Drawing for the job (mm, zero at the part's lowest x, y, z). Coordinates: 2 decimals unless noted, no trailing zeros. Write each loop counter-clockwise with the first axis right and the second up, starting at its lowest first coordinate (ties: lowest second). Pieces come first, ordered by that corner, then holes. Notation, with made-up numbers: M 52.5,69 L 75.5,69 A25 cw 75.5,84 Z; hole C 23,35 d1. An arc over 180 degrees is marked long. Put each result on its own line as item: value. Start each with the question number.
Q1. Drill centre lines: line 1 along X through (y, z) = (14.5, 0.7) (3 decimals); line 2 along Y through (x, z) = (20, 0.45); line 3 along Y through (x, z) = (30.5, 0.7). Where is each one in solid material? Low to high.
Q2. Cut at D-D (x = 23.5). Write the cut outline in (y, z), then the cut area to 3 significant figures.
Q3. Cut at C-C (x = 12.5). Write the cut outline in (y, z), then the cut area to 3 significant figures.
Q4. Cut at B-B (z = 0.35). Write the cut outline in (x, y) (3 decimals).
Q5. Cut at A-A (y = 21.5). Write the cut outline in (x, z) (3 decimals), then the cut area to 4 significant figures.
Q6. Drop flat-ended pins along their axis: pin 1 (0.8 mm diameter, centred on y = 15, z = 1, fed in from +X); pin 2 (0.8 mm diameter, centred on x = 40, z = 0.5, fed in from -Y). Give the stop position or say it passes through.
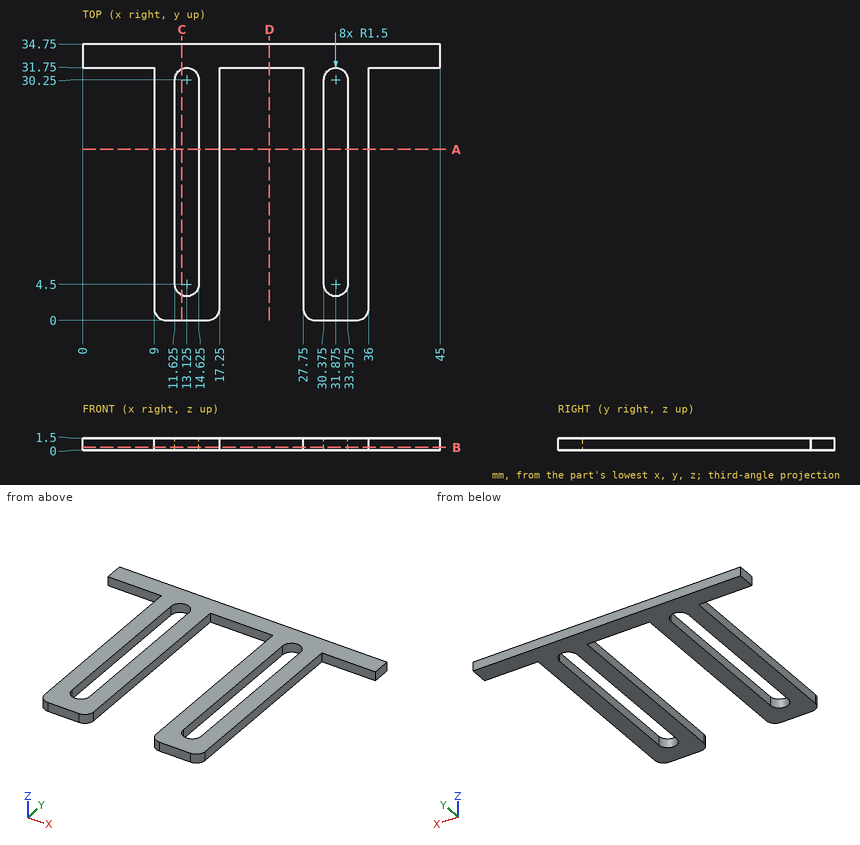
Computed values:
1. line 1: 9 to 11.625, 14.625 to 17.25, 27.75 to 30.375, 33.375 to 36
1. line 2: 31.75 to 34.75
1. line 3: 0 to 3.9, 30.85 to 34.75
2. outline: M 31.75,0 L 34.75,0 L 34.75,1.5 L 31.75,1.5 Z
2. area: 4.50 mm2
3. outline: M 0,0 L 3.14,0 L 3.14,1.5 L 0,1.5 Z; M 31.61,0 L 34.75,0 L 34.75,1.5 L 31.61,1.5 Z
3. area: 9.41 mm2
4. outline: M 0,31.75 L 9,31.75 L 9,1.5 A1.5 ccw 10.5,0 L 15.75,0 A1.5 ccw 17.25,1.5 L 17.25,31.75 L 27.75,31.75 L 27.75,1.5 A1.5 ccw 29.25,0 L 34.5,0 A1.5 ccw 36,1.5 L 36,31.75 L 45,31.75 L 45,34.75 L 0,34.75 Z; hole M 11.625,4.5 A1.5 ccw 14.625,4.5 L 14.625,30.25 A1.5 ccw 11.625,30.25 Z; hole M 30.375,4.5 A1.5 ccw 33.375,4.5 L 33.375,30.25 A1.5 ccw 30.375,30.25 Z
5. outline: M 9,0 L 11.625,0 L 11.625,1.5 L 9,1.5 Z; M 14.625,0 L 17.25,0 L 17.25,1.5 L 14.625,1.5 Z; M 27.75,0 L 30.375,0 L 30.375,1.5 L 27.75,1.5 Z; M 33.375,0 L 36,0 L 36,1.5 L 33.375,1.5 Z
5. area: 15.75 mm2
6. pin 1: x = 36
6. pin 2: y = 31.75
